from build123d import *

# Parameters (mm, degrees)
SALIENTE_EXTRUIR1_DEPTH = 8
CROQUIS2_R              = 2.38125
CORTAR_EXTRUIR1_DEPTH   = 16
REDONDEO1_R             = 3


with BuildPart() as part:
    # Croquis1 → Saliente-Extruir1 (new, symmetric)
    with BuildSketch(Plane.XY):
        with BuildLine():
            Line((25.5, -1.5), (18.740064034, -1.5))
            ThreePointArc((18.740064034, -1.5), (18.361312119, -4.037600434), (17.640578222, -6.5))
            Line((17.640578222, -6.5), (25.5, -6.5))
            Line((25.5, -6.5), (25.5, -1.5))
        make_face()
        with BuildLine():
            Line((18.740064034, -1.5), (14.924811557, -1.5))
            ThreePointArc((14.924811557, -1.5), (14.43972216, -4.06133278), (13.518505835, -6.5))
            Line((13.518505835, -6.5), (17.640578222, -6.5))
            ThreePointArc((17.640578222, -6.5), (18.361312119, -4.037600434), (18.740064034, -1.5))
        make_face()
        with BuildLine():
            ThreePointArc((13.518505835, -6.5), (0, -15), (-13.518505835, -6.5))
            Line((-13.518505835, -6.5), (-17.640578222, -6.5))
            ThreePointArc((-17.640578222, -6.5), (0, -18.8), (17.640578222, -6.5))
            Line((17.640578222, -6.5), (13.518505835, -6.5))
        make_face()
        with BuildLine():
            ThreePointArc((-13.518505835, -6.5), (-14.43972216, -4.06133278), (-14.924811557, -1.5))
            Line((-14.924811557, -1.5), (-18.740064034, -1.5))
            ThreePointArc((-18.740064034, -1.5), (-18.361312119, -4.037600434), (-17.640578222, -6.5))
            Line((-17.640578222, -6.5), (-13.518505835, -6.5))
        make_face()
        with BuildLine():
            ThreePointArc((-17.640578222, -6.5), (-18.361312119, -4.037600434), (-18.740064034, -1.5))
            Line((-18.740064034, -1.5), (-25.5, -1.5))
            Line((-25.5, -1.5), (-25.5, -6.5))
            Line((-25.5, -6.5), (-17.640578222, -6.5))
        make_face()
    extrude(amount=SALIENTE_EXTRUIR1_DEPTH, both=True)

    # Croquis2 → Cortar-Extruir1 (cut)
    with BuildSketch(Plane(origin=(0, -1.5, 0), x_dir=(1, 0, 0), z_dir=(0, 1, 0))):
        with Locations(Location((-21.5, 0, 0), (0, 0, 180))):
            Circle(CROQUIS2_R)
        with Locations(Location((21.5, 0, 0), (0, 0, 180))):
            Circle(CROQUIS2_R)
    extrude(amount=-CORTAR_EXTRUIR1_DEPTH, mode=Mode.SUBTRACT)

    # Redondeo1
    redondeo1_edges = [part.edges().sort_by_distance(p)[0] for p in [
        (25.5, -4, -8),
        (-25.5, -4, -8),
        (-14.924811557, -1.5, 0),
        (14.924811557, -1.5, 0),
        (-25.5, -4, 8),
        (25.5, -4, 8),
    ]]
    fillet(redondeo1_edges, radius=REDONDEO1_R)


solid = part.part
The listing builds one solid part. Answer for the finished solid, in the listing's coordinates (mm). A direction names the side the tool comes from. Coordinates: 2 decimals unless noted, no trailing zeros. Loops run counter-clockwise (first coordinate to the right, second up) from the corner with the lowest first, then second, coordinate; pieces in that order, holes last. Notation, with made-up numbers: (-34.75, -23) -> (-29.75, -23) arc R26 cw to (-29.75, 10) -> close; hole circle Ø11 at (41.5, 69.5). An arc over 180 degrees is marked (long way). Answer in a Markdown table with one row per item. Add a question column.
1. Consider line 1 (Z direction, x = -21.5, y = -3.85); line 2 (Y direction, x = 18.5, z = -3.25); line 3 (X direction, y = -3.25, z = 3.25). Determine where each line is inside the solid, lowest interval first. Write a range as [from, to].
2. The part is cut by section C-C, the plane z = -3. Write down the section's boundary in (x, y).
3. For faces 1 (the cylindrical face through (15.613, -2.111, 0.112)), 2 (the flat face through (-23.4, -6.5, 1.9)), 3 (the cylindrical face through (-0.32, -18.797, 0.112)), 4 (the cylindrical face through (-23.77, -3.96, 0.72)), 5 (the flat face through (19.8, -6.5, 1.9)), determine the directions among +Z, -Z, +X, -X, +Y, -Y from which every point of the face is accessible in a straight line to the end or side of a thin tool.
4. Determine the mould class of faces 6 (the cylindrical face through (24.6, -3.96, -7.14)), 7 (the flat face through (-1.8, -15.2, -8)), 8 (the cylindrical face through (19.23, -3.96, 0.72)) for opening direction X: +X half, -X half, draft (parallel to the pull), parting line (faces both ways), or undercut.
5. The part is cut by section D-D, the plane y = -13. Write down the section's boundary in (x, z), then the cut area to 3 significant figures.
6. The part is cut by section B-B, the plane z = 0. Write down the section's boundary in (x, y), then the cut area to 3 significant figures.
7. The part is cut by section A-A, the plane x = -21.5. Write down the section's boundary in (y, z), then the cut area to 3 significant figures.
8. Flat-ended cylindrical pins translate along their axes: P1, Ø2, axis at y = -14, z = 0.5, coming from the +X side; P2, Ø1, axis at x = 13.5, z = 5, coming from the -Y side; P3, Ø3, axis at x = 21.5, z = 0, coming from the -Y side; P4, Ø8.5, axis at x = 20.5, z = 2, coming from the -Y side. Find the tip coordinate at first contact, or state that the pin passes through.
Answer below:
| question | item | result |
|---|---|---|
| 1 | line 1 | [-8, -2.38], [2.38, 8] |
| 1 | line 2 | [-6.5, -1.5] |
| 1 | line 3 | [-25.5, -14.7], [14.7, 25.5] |
| 2 | outline | (-25.5, -6.5) -> (-17.64, -6.5) arc R18.8 ccw to (17.64, -6.5) -> (25.5, -6.5) -> (25.5, -1.5) -> (17.43, -1.5) arc R3 ccw to (14.52, -3.75) arc R15 cw to (-14.52, -3.75) arc R3 ccw to (-17.43, -1.5) -> (-25.5, -1.5) -> close |
| 3 | face 1 | +Z, -Z, +Y |
| 3 | face 2 | +Z, -Z, -X, -Y |
| 3 | face 3 | +Z, -Z, -Y |
| 3 | face 4 | +Y, -Y |
| 3 | face 5 | +Z, -Z, +X, -Y |
| 4 | face 6 | +X half |
| 4 | face 7 | draft |
| 4 | face 8 | undercut |
| 5 | outline | (-13.58, -8) -> (-7.48, -8) -> (-7.48, 8) -> (-13.58, 8) -> close; (7.48, -8) -> (13.58, -8) -> (13.58, 8) -> (7.48, 8) -> close |
| 5 | area | 195 mm2 |
| 6 | outline | (-25.5, -6.5) -> (-23.88, -6.5) -> (-23.88, -1.5) -> (-25.5, -1.5) -> close; (-19.12, -6.5) -> (-17.64, -6.5) arc R18.8 ccw to (17.64, -6.5) -> (19.12, -6.5) -> (19.12, -1.5) -> (17.43, -1.5) arc R3 ccw to (14.52, -3.75) arc R15 cw to (-14.52, -3.75) arc R3 ccw to (-17.43, -1.5) -> (-19.12, -1.5) -> close; (23.88, -6.5) -> (25.5, -6.5) -> (25.5, -1.5) -> (23.88, -1.5) -> close |
| 6 | area | 212 mm2 |
| 7 | outline | (-6.5, -8) -> (-1.5, -8) -> (-1.5, -2.38) -> (-6.5, -2.38) -> close; (-6.5, 2.38) -> (-1.5, 2.38) -> (-1.5, 8) -> (-6.5, 8) -> close |
| 7 | area | 56.2 mm2 |
| 8 | P1 | x = 13.58 |
| 8 | P2 | y = -13.58 |
| 8 | P3 | through |
| 8 | P4 | y = -9.45 |
